Autodesk Inventor part; units mm, degrees
ref_plane "YZ Plane" through (0, 0, 0) normal (1, 0, 0) x (0, 1, 0)
ref_plane "XZ Plane" through (0, 0, 0) normal (0, 1, 0) x (-1, 0, 0)
ref_plane "XY Plane" through (0, 0, 0) normal (0, 0, 1) x (1, 0, 0)
sketch "Sketch3" plane through (0, 0, 0) normal (1, 0, 0) x (0, 1, 0)
  line L0 (0, 0) -> (80, 0)
  line L1 (80, 0) -> (80, 73)
  line L2 (80, 73) -> (0, 73)
  line L3 (0, 73) -> (0, 0)
  dimension "d8" = 80
  dimension "d9" = 73
extrude "Extrusion3" add sketch "Sketch3" along normal blind 40
shell "Shell1" thickness 1 removed faces 3 at (26.6667, 0, 48.6667) at (0, 53.3333, 24.3333) at (40, 53.3333, 24.3333)
sketch "Sketch4" plane through (0, 0, 73) normal (0, 0, 1) x (1, 0, 0)
  line L0 (0, 0) -> (40, 0)
  line L1 (0, 80) -> (40, 80)
  circle A0 centre (20, 8.0945) radius 2
  dimension "d13" = 4
extrude "Extrusion4" cut sketch "Sketch4" against normal blind 1
sketch "Sketch5" plane through (0, 0, 73) normal (0, 0, 1) x (1, 0, 0)
  line L0 (0, 80) -> (40, 80)
  circle A0 centre (20, 67.4876) radius 3.5
  point P0 (0, 0)
  dimension "d16" = 7
extrude "Extrusion5" cut sketch "Sketch5" against normal blind 1
properties part number "MAN_BASIS_THIRD_STRUCTURE" material "ABS Plastic"
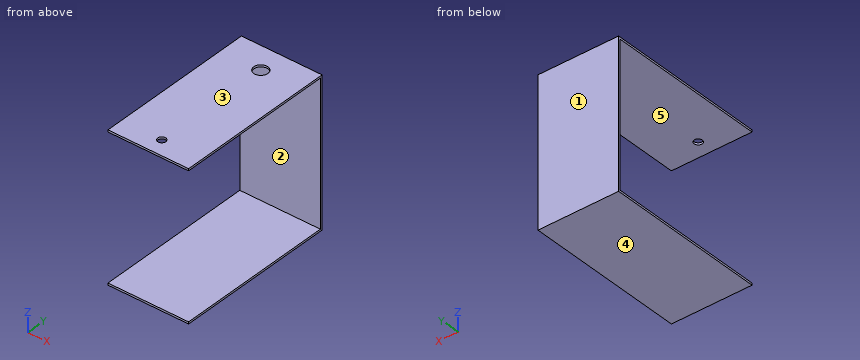
Read the model definition and answer for the solid it produces. Units are mm, in the model's axes. Face numbers are marked on the shaded views. A direction names the side the tool comes from. Round coordinates to 2 decimals unless told otherwise and drop trailing zeros. Write each loop counter-clockwise with the first axis right and the second up, starting at its lowest first coordinate (ties: lowest second). Pieces come first, ordered by that corner, then holes. Notation, with made-up numbers: M -16,4 L 28,4 A13 ccw 28,29 Z; hole C -10.75,-13.5 d3. An arc over 180 degrees is marked long. One line per item, written item: value.
Q1. Find section A-A on y = 17. Write down the section's boundary in (x, z).
Data:
outline: M 0,0 L 40,0 L 40,1 L 0,1 Z; M 0,72 L 40,72 L 40,73 L 0,73 Z
Q2. Find section C-C on x = 30. Write down the section's boundary in (y, z), plus the area to 3 significant figures.
Data:
outline: M 0,0 L 80,0 L 80,73 L 0,73 L 0,72 L 79,72 L 79,1 L 0,1 Z
area: 231 mm2
Q3. Find section D-D on z = 27.5. Write down the section's boundary in (x, y).
Data:
outline: M 0,79 L 40,79 L 40,80 L 0,80 Z
Q4. Flat-ended cylindrical pins translate along their axes: pin 1 Ø10 at (y, z) = (62.5, 63.5) entering from +X; pin 2 Ø3 at (x, y) = (20, 8.09) entering from -Z; pin 3 Ø12 at (x, z) = (24, 31) entering from -Y. Find the tip coordinate at first contact, or state that the pin passes through.
Data:
pin 1: through
pin 2: z = 0
pin 3: y = 79
Q5. Which of the six approach directions +Z, -Z, +X, -X, +Y, -Y give full straight-line access (tool end or side, diameter ignored) to the marked faces 4 and 5?
Data:
face 4: -Z, +X, -X, +Y, -Y
face 5: +X, -X, -Y
Q6. For a pull along Z with two mould halves and no side action, classify the marked faces 1, 2 and 3 as +Z half, -Z half, draft (parallel to the pull), parting line (faces both ways), or undercut.
Data:
face 1: draft
face 2: undercut
face 3: +Z half
Q7. Straight lines are drawn through the part: line 1 (Y direction, x = 20, z = 72.3); line 2 (Z direction, x = 23.5, y = 17); line 3 (Y direction, x = 38.5, z = 56). For each, find the intervals that lie inside material, in ascending order. Write a range as [from, to].
Data:
line 1: [0, 6.09], [10.09, 63.99], [70.99, 80]
line 2: [0, 1], [72, 73]
line 3: [79, 80]
Q8. Find section B-B on x = 20. Write down the section's boundary in (y, z).
Data:
outline: M 0,0 L 80,0 L 80,73 L 70.99,73 L 70.99,72 L 79,72 L 79,1 L 0,1 Z; M 0,72 L 6.09,72 L 6.09,73 L 0,73 Z; M 10.09,72 L 63.99,72 L 63.99,73 L 10.09,73 Z
